Here's how the part is built. I have some questions about the finished solid (model axes, mm). A direction names the side the tool comes from. Give positions to 0.01 mm unless a question says otherwise; leave off trailing zeros. Loops run counter-clockwise (first coordinate to the right, second up) from the corner with the lowest first, then second, coordinate; pieces in that order, holes last. Notation, with made-up numbers: (-39.75, 14) - (-35.75, 14) arc R32 cw to (-35.75, 48) - close; hole circle Ø3 at (-2.5, 22). An arc over 180 degrees is marked (long way). Return JSON: item names as keys, results as strings. Group by question number.
(1) For P1, Ø1, axis at x = 23, y = 1, coming from the +Z side; P2, Ø1.9, axis at x = -32.5, z = 0, coming from the -Y side; P3, Ø0.5, axis at x = -32, y = 0.5, coming from the +Z side, each with a flat end and sliding along its axis, tell me the tip position at first contact or that it passes through.
(2) If we section it at B-B (z = 0): Please give me the cut outline in (x, y).
(3) I need wall thicknesses on probe 1 along Z at (x, y) = (27, 0.35); probe 2 along Z at (x, y) = (21.5, 1.9); probe 3 along X at (y, z) = (0.25, 16). Which ranges of each line are inside material? Lowest first, please. Write a range as [from, to].
(4) If we mould it in two halves opening along Z, with no side actions, what happens to faces 4 (the flat face through (0, 1, 11.35)), 5 (the flat face through (36.5, 1, 0)), 6 (the cylindrical face through (36.344, 1.014, -13.797))? For each: released by +Z, released by -Z, zero draft, split by the parting line, or undercut.
(5) On a 3-axis mill with a long thin cutter (end or side, diameter ignored), from which of +Z, -Z, +X, -X, +Y, -Y can I reach the whole of each face in a straight line? I mean faces 1 (the cylindrical face through (-30.47, 0.99, 17.16)), 2 (the flat face through (-20, 1, -11.35)), 3 (the flat face through (34.66, 0.99, -15.69)). Say none if no direction works.
(6) If we section it at C-C (y = 0.4): State how many separate pieces and enclosed holes the cut face has, then the cut area to 3 significant figures.
(7) If we section it at A-A (x = -17): Please give me the cut outline in (y, z).
```python
from build123d import *

# Parameters (mm, degrees)
SKETCH_1_W          = 73
SKETCH_1_H          = 37.7
SKETCH_1_R          = 1.6
EXTRUDE_1_DEPTH     = 2
SKETCH_2_W          = 59
SKETCH_2_H          = 22.7
CUT_EXTRUDE_1_DEPTH = 10
SKETCH_3_W          = 59
SKETCH_3_H          = 4
EXTRUDE_1_2_DEPTH   = 2
CUT_EXTRUDE_START   = -2
SKETCH_4_R          = 1.6
CUT_EXTRUDE_2_DEPTH = 2
FILLET_2_R          = 1.5
CHAMFER_1_SIZE      = 5
SKETCH_6_R          = 3
CUT_EXTRUDE_3_DEPTH = 10
CUT_EXTRUDE_4_DEPTH = 10
FILLET_3_R          = 2


with BuildPart() as part:
    # 草图1 → Extrude 1 (new body)
    with BuildSketch(Plane(origin=(0, 0, 0), x_dir=(1, 0, 0), z_dir=(0, 1, 0))):
        Rectangle(SKETCH_1_W, SKETCH_1_H)
        with Locations(Location((10, -14.35, 0), (0, 0, 270))):
            Circle(SKETCH_1_R, mode=Mode.SUBTRACT)
        with Locations(Location((-10, -14.35, 0), (0, 0, 270))):
            Circle(SKETCH_1_R, mode=Mode.SUBTRACT)
        with Locations(Location((-10, 14.35, 0), (0, 0, 270))):
            Circle(SKETCH_1_R, mode=Mode.SUBTRACT)
        with Locations(Location((10, 14.35, 0), (0, 0, 270))):
            Circle(SKETCH_1_R, mode=Mode.SUBTRACT)
        with Locations(Location((-32.5, 0, 0), (0, 0, 270))):
            Circle(SKETCH_1_R, mode=Mode.SUBTRACT)
        with Locations(Location((32.5, 0, 0), (0, 0, 270))):
            Circle(SKETCH_1_R, mode=Mode.SUBTRACT)
    extrude(amount=EXTRUDE_1_DEPTH)

    # 草图2 → 切除-拉伸1 (cut)
    with BuildSketch(Plane(origin=(0, 2, 0), x_dir=(1, 0, 0), z_dir=(0, 1, 0))):
        Rectangle(SKETCH_2_W, SKETCH_2_H)
    extrude(amount=-CUT_EXTRUDE_1_DEPTH, mode=Mode.SUBTRACT)

    # 草图3 → Extrude 1 2 (add)
    with BuildSketch(Plane(origin=(0, 2, 0), x_dir=(1, 0, 0), z_dir=(0, 1, 0))):
        Rectangle(SKETCH_3_W, SKETCH_3_H)
        Polygon((-11.640877602, 13.206531288), (8.359122398, -15.493468712), (11.640877602, -13.206531288), (-8.359122398, 15.493468712), align=None)
        Polygon((8.359122398, 15.493468712), (-11.640877602, -13.206531288), (-8.359122398, -15.493468712), (11.640877602, 13.206531288), align=None)
    extrude(amount=-EXTRUDE_1_2_DEPTH)

    # 草图4 → 切除-拉伸2 (cut)
    with BuildSketch(Plane(origin=(0, 2, 0), x_dir=(1, 0, 0), z_dir=(0, 1, 0)).offset(CUT_EXTRUDE_START)):
        with Locations(Location((10, -14.35, 0), (0, 0, 270))):
            Circle(SKETCH_4_R)
        with Locations(Location((-10, -14.35, 0), (0, 0, 270))):
            Circle(SKETCH_4_R)
        with Locations(Location((10, 14.35, 0), (0, 0, 270))):
            Circle(SKETCH_4_R)
        with Locations(Location((-10, 14.35, 0), (0, 0, 270))):
            Circle(SKETCH_4_R)
    extrude(amount=CUT_EXTRUDE_2_DEPTH, mode=Mode.SUBTRACT)

    # 圆角2
    fillet_2_edges = [part.edges().sort_by_distance(p)[0] for p in [
        (-3.831448133, 1, 2),
        (0, 1, -3.498128071),
        (3.831448133, 1, -2),
        (3.831448133, 1, 2),
        (29.5, 1, 2),
        (-29.5, 1, 2),
        (-3.831448133, 1, -2),
        (-29.5, 1, -2),
        (29.5, 1, -2),
        (29.5, 1, -11.35),
        (29.5, 1, 11.35),
        (-29.5, 1, 11.35),
        (-29.5, 1, -11.35),
        (-10.347127575, 1, -11.35),
        (10.347127575, 1, -11.35),
        (5.471687756, 1, -11.35),
        (-5.471687756, 1, -11.35),
        (-5.471687756, 1, 11.35),
        (-10.347127575, 1, 11.35),
        (10.347127575, 1, 11.35),
        (5.471687756, 1, 11.35),
        (0, 1, 3.498128071),
    ]]
    fillet(fillet_2_edges, radius=FILLET_2_R)

    # 倒角1
    chamfer_1_edges = [part.edges().sort_by_distance(p)[0] for p in [
        (36.5, 1, 18.85),
        (-36.5, 1, 18.85),
        (-36.5, 1, -18.85),
        (36.5, 1, -18.85),
    ]]
    chamfer(chamfer_1_edges, length=CHAMFER_1_SIZE)

    # 草图6 → 切除-拉伸3 (cut)
    with BuildSketch(Plane(origin=(0, 2, 0), x_dir=(1, 0, 0), z_dir=(0, 1, 0))):
        with Locations((27, 17.5)):
            Circle(SKETCH_6_R)
        with Locations((27, -17.5)):
            Circle(SKETCH_6_R)
        with Locations((-27, -17.5)):
            Circle(SKETCH_6_R)
        with Locations((-27, 17.5)):
            Circle(SKETCH_6_R)
    extrude(amount=-CUT_EXTRUDE_3_DEPTH, mode=Mode.SUBTRACT)

    # 草图7 → 切除-拉伸4 (cut)
    with BuildSketch(Plane(origin=(0, 2, 0), x_dir=(1, 0, 0), z_dir=(0, 1, 0))):
        with BuildLine():
            Line((30, -17.5), (32.85, -17.5))
            Line((32.85, -17.5), (31.5, -18.85))
            Line((31.5, -18.85), (29.679085665, -18.85))
            ThreePointArc((29.679085665, -18.85), (29.91866896, -18.193809414), (30, -17.5))
        make_face()
        with BuildLine():
            Line((24, -17.5), (24, -18.85))
            Line((24, -18.85), (24.320914335, -18.85))
            ThreePointArc((24.320914335, -18.85), (24.08133104, -18.193809414), (24, -17.5))
        make_face()
        with BuildLine():
            Line((24.320914335, 18.85), (24, 18.85))
            Line((24, 18.85), (24, 17.5))
            ThreePointArc((24, 17.5), (24.08133104, 18.193809414), (24.320914335, 18.85))
        make_face()
        with BuildLine():
            Line((31.5, 18.85), (32.85, 17.5))
            Line((32.85, 17.5), (30, 17.5))
            ThreePointArc((30, 17.5), (29.91866896, 18.193809414), (29.679085665, 18.85))
            Line((29.679085665, 18.85), (31.5, 18.85))
        make_face()
        with BuildLine():
            Line((-30, 17.5), (-32.85, 17.5))
            Line((-32.85, 17.5), (-31.5, 18.85))
            Line((-31.5, 18.85), (-29.679085665, 18.85))
            ThreePointArc((-29.679085665, 18.85), (-29.91866896, 18.193809414), (-30, 17.5))
        make_face()
        with BuildLine():
            Line((-24, 17.5), (-24, 18.85))
            Line((-24, 18.85), (-24.320914335, 18.85))
            ThreePointArc((-24.320914335, 18.85), (-24.08133104, 18.193809414), (-24, 17.5))
        make_face()
        with BuildLine():
            Line((-24.320914335, -18.85), (-24, -18.85))
            Line((-24, -18.85), (-24, -17.5))
            ThreePointArc((-24, -17.5), (-24.08133104, -18.193809414), (-24.320914335, -18.85))
        make_face()
        with BuildLine():
            Line((-31.5, -18.85), (-32.85, -17.5))
            Line((-32.85, -17.5), (-30, -17.5))
            ThreePointArc((-30, -17.5), (-29.91866896, -18.193809414), (-29.679085665, -18.85))
            Line((-29.679085665, -18.85), (-31.5, -18.85))
        make_face()
    extrude(amount=-CUT_EXTRUDE_4_DEPTH, mode=Mode.SUBTRACT)

    # 圆角3
    fillet_3_edges = [part.edges().sort_by_distance(p)[0] for p in [
        (-36.5, 1, -13.85),
        (-36.5, 1, 13.85),
        (36.5, 1, 13.85),
        (36.5, 1, -13.85),
        (-32.85, 1, 17.5),
        (-30, 1, 17.5),
        (24, 1, 18.85),
        (30, 1, 17.5),
        (32.85, 1, 17.5),
        (32.85, 1, -17.5),
        (30, 1, -17.5),
        (24, 1, -18.85),
        (-24, 1, -18.85),
        (-30, 1, -17.5),
        (-32.85, 1, -17.5),
        (-24, 1, 18.85),
    ]]
    fillet(fillet_3_edges, radius=FILLET_3_R)


solid = part.part
```
Values:
{
 "1": {"P1": "z = 18.8", "P2": "through", "P3": "z = 17.5"},
 "2": {"outline": "(-36.5, 0) - (-34.1, 0) - (-34.1, 2) - (-36.5, 2) - close; (-30.9, 0) - (30.9, 0) - (30.9, 2) - (-30.9, 2) - close; (34.1, 0) - (36.5, 0) - (36.5, 2) - (34.1, 2) - close"},
 "3": {"probe 1": "[-14.5, -11.35], [-2, 2], [11.35, 14.5]", "probe 2": "[-18.85, -11.35], [-2, 2], [11.35, 18.85]", "probe 3": "[-34.35, -29.6], [-24.4, 24.4], [29.6, 34.35]"},
 "4": {"face 4": "undercut", "face 5": "zero draft", "face 6": "released by -Z"},
 "5": {"face 1": "+Z, +Y, -Y", "face 2": "+Y, -Y", "face 3": "-Z, +X, +Y, -Y"},
 "6": {"separate pieces": "1", "enclosed holes": "12", "area": "1,640 mm2"},
 "7": {"outline": "(0, -18.85) - (2, -18.85) - (2, -11.35) - (0, -11.35) - close; (0, -2) - (2, -2) - (2, 2) - (0, 2) - close; (0, 11.35) - (2, 11.35) - (2, 18.85) - (0, 18.85) - close"}
}
